from build123d import *

# Parameters (mm, degrees)
SKETCH1_R           = 11
SKETCH1_R_2         = 3.142556432
SKETCH1_R_3         = 22.5
SKETCH1_R_4         = 3
BOSS_EXTRUDE1_DEPTH = 15
BOSS_EXTRUDE2_START = 10
SKETCH3_R           = 11
SKETCH3_R_2         = 4.25
BOSS_EXTRUDE2_DEPTH = 10


with BuildPart() as part:
    # Sketch1 → Boss-Extrude1 (new body)
    with BuildSketch(Plane.XY):
        with BuildLine():
            Line((-120, 172.705707432), (135, 172.705707432))
            ThreePointArc((135, 172.705707432), (170.355339059, 158.061046491), (185, 122.705707432))
            Line((185, 122.705707432), (185, 112.705707432))
            Line((185, 112.705707432), (170, 112.705707432))
            Line((170, 112.705707432), (170, 82.705707432))
            Line((170, 82.705707432), (185, 82.705707432))
            Line((185, 82.705707432), (185, 52.705707432))
            Line((185, 52.705707432), (170, 52.705707432))
            Line((170, 52.705707432), (170, 22.705707432))
            Line((170, 22.705707432), (185, 22.705707432))
            Line((185, 22.705707432), (185, -7.294292568))
            Line((185, -7.294292568), (170, -7.294292568))
            Line((170, -7.294292568), (170, -117.094321696))
            Line((170, -117.094321696), (185, -117.094321696))
            Line((185, -117.094321696), (185, -147.094321696))
            Line((185, -147.094321696), (170, -147.094321696))
            Line((170, -147.094321696), (170, -162.094292568))
            Line((170, -162.094292568), (170, -177.170123414))
            Line((170, -177.170123414), (140, -177.170123414))
            Line((140, -177.170123414), (140, -162.094292568))
            Line((140, -162.094292568), (110, -162.094292568))
            Line((110, -162.094292568), (110, -177.182197899))
            Line((110, -177.182197899), (80, -177.182197899))
            Line((80, -177.182197899), (80, -162.094292568))
            Line((80, -162.094292568), (50, -162.094292568))
            Line((50, -162.094292568), (50, -177.165057848))
            Line((50, -177.165057848), (20, -177.165057848))
            Line((20, -177.165057848), (20, -162.094292568))
            Line((20, -162.094292568), (-20, -162.094292568))
            Line((-20, -162.094292568), (-20, -176.865618337))
            Line((-20, -176.865618337), (-50, -176.865618337))
            Line((-50, -176.865618337), (-50, -162.094292568))
            Line((-50, -162.094292568), (-80, -162.094292568))
            Line((-80, -162.094292568), (-80, -177.034188853))
            Line((-80, -177.034188853), (-110, -177.034188853))
            Line((-110, -177.034188853), (-110, -162.094292568))
            Line((-110, -162.094292568), (-140, -162.094292568))
            Line((-140, -162.094292568), (-140, -176.801614054))
            Line((-140, -176.801614054), (-170, -176.801614054))
            Line((-170, -176.801614054), (-170, -167.294292568))
            Line((-170, -167.294292568), (-170, 122.705707432))
            ThreePointArc((-170, 122.705707432), (-155.355339059, 158.061046491), (-120, 172.705707432))
        make_face()
        with Locations((145, -107)):
            Circle(SKETCH1_R, mode=Mode.SUBTRACT)
        with Locations((-131.5, 98.85)):
            Circle(SKETCH1_R_2, mode=Mode.SUBTRACT)
        with Locations((-81, 98.85)):
            Circle(SKETCH1_R_3, mode=Mode.SUBTRACT)
        with Locations((-61.5, 65.075009252)):
            Circle(SKETCH1_R_4, mode=Mode.SUBTRACT)
        with Locations((-61.5, 132.624990748)):
            Circle(SKETCH1_R_4, mode=Mode.SUBTRACT)
        with BuildLine():
            Line((-55.995398281, -49.8), (-55.995398281, -99.8))
            ThreePointArc((-55.995398281, -99.8), (-0.995398281, -151.720675316), (54.004601719, -99.8))
            Line((54.004601719, -99.8), (54.004601719, -49.8))
            ThreePointArc((54.004601719, -49.8), (43.536944591, -20.017496175), (14.731892041, -7.100905005))
            Line((14.731892041, -7.100905005), (-16.722688603, -7.100905005))
            ThreePointArc((-16.722688603, -7.100905005), (-45.527741152, -20.017496175), (-55.995398281, -49.8))
        make_face(mode=Mode.SUBTRACT)
    extrude(amount=BOSS_EXTRUDE1_DEPTH)

    # Sketch3 → Boss-Extrude2 (add)
    with BuildSketch(Plane(origin=(0, 0, 17), x_dir=(-1, 0, 0), z_dir=(0, 0, -1)).offset(BOSS_EXTRUDE2_START)):
        with Locations((-145, -107)):
            Circle(SKETCH3_R)
        with Locations((-145, -107)):
            Circle(SKETCH3_R_2, mode=Mode.SUBTRACT)
    extrude(amount=-BOSS_EXTRUDE2_DEPTH)


solid = part.part
For this review, take the finished solid that the model builds, in its own axes (mm). A direction names the side the tool comes from. Round coordinates to 2 decimals unless told otherwise and drop trailing zeros. Loops run counter-clockwise (first coordinate to the right, second up) from the corner with the lowest first, then second, coordinate; pieces in that order, holes last. Notation, with made-up numbers: (-31.5, 52.5) - (-2.5, 52.5) arc R17 ccw to (-2.5, 76.5) - close; hole circle Ø4 at (31.25, 21.25). An arc over 180 degrees is marked (long way). Use one line per item in the form item = value.
Item 1: For line 1 (X direction, y = -59, z = 12.5); line 2 (X direction, y = 101.5, z = 6.75); line 3 (X direction, y = -107, z = 3), list the stretches that pass through material, from the lowest coordinate up.
Answers:
line_1 = -170 to -56, 54 to 170
line_2 = -170 to -133.19, -129.81 to -103.34, -58.66 to 170
line_3 = -170 to -55.1, 53.11 to 134, 156 to 170
Item 2: Mouldability with a two-part tool opening along X and no side actions: class faces 4 (the cylindrical face through (-45.218, -19.685, 7.395)), 5 (the cylindrical face through (43.84, -20.35, 7.4)), 6 (the flat face through (185, 118, 7)), 7 (the flat face through (178, 52.706, 7)) as +X half, -X half, draft (parallel to the pull), parting line (faces both ways), or undercut.
Answers:
face_4 = undercut
face_5 = undercut
face_6 = +X half
face_7 = draft
Item 3: Consider section A-A on y = -12. Write out the cut boundary in (x, z).
Answers:
outline = (-170, 0) - (-35.28, 0) - (-35.28, 15) - (-170, 15) - close; (33.29, 0) - (170, 0) - (170, 15) - (33.29, 15) - close
Item 4: Consider section C-C on y = -107. Write out the cut boundary in (x, z), then the cut area to 3 significant figures.
Answers:
outline = (-170, 0) - (-55.1, 0) - (-55.1, 15) - (-170, 15) - close; (53.11, 0) - (134, 0) - (134, 7) - (140.75, 7) - (140.75, 17) - (134, 17) - (134, 15) - (53.11, 15) - close; (149.25, 7) - (156, 7) - (156, 0) - (170, 0) - (170, 15) - (156, 15) - (156, 17) - (149.25, 17) - close
area = 3,280 mm^2
Item 5: Consider section B-B on x = 145. Write out the cut boundary in (y, z), then the cut area to 3 significant figures.
Answers:
outline = (-177.17, 0) - (-118, 0) - (-118, 7) - (-111.25, 7) - (-111.25, 17) - (-118, 17) - (-118, 15) - (-177.17, 15) - close; (-102.75, 7) - (-96, 7) - (-96, 0) - (171.7, 0) - (171.7, 15) - (-96, 15) - (-96, 17) - (-102.75, 17) - close
area = 5,040 mm^2
Item 6: Tool access review of faces 1 (the flat face through (0, -162.094, 7)), 2 (the flat face through (170, -162, 7)), 3 (the flat face through (-155, -176.802, 7)): name each direction out of +Z, -Z, +X, -X, +Y, -Y from which nothing blocks a thin tool from reaching the whole face with its end or side.
Answers:
face_1 = +Z, -Z, -Y
face_2 = +Z, -Z, +X, -Y
face_3 = +Z, -Z, -X, -Y
Item 7: Consider section D-D on z = 10.5. State how many separate pieces and enclosed holes the cut face has, then the cut area to 3 significant figures.
Answers:
separate_pieces = 1
enclosed_holes = 6
area = 102,000 mm^2
Item 8: Clearance check with flat-ended pins moving along their axes: P1, Ø4.5, axis at y = 31.5, z = 4.5, coming from the +X side; P2, Ø7.5, axis at x = -123.5, z = 7, coming from the -Y side; P3, Ø7.5, axis at x = 176, z = 8, coming from the -Y side; P4, Ø4, axis at x = -131.5, y = 98.85, coming from the +Z side. State where each tip first meets the part, or that it passes through.
Answers:
P1 = 170
P2 = -162.09
P3 = -147.09
P4 = through
